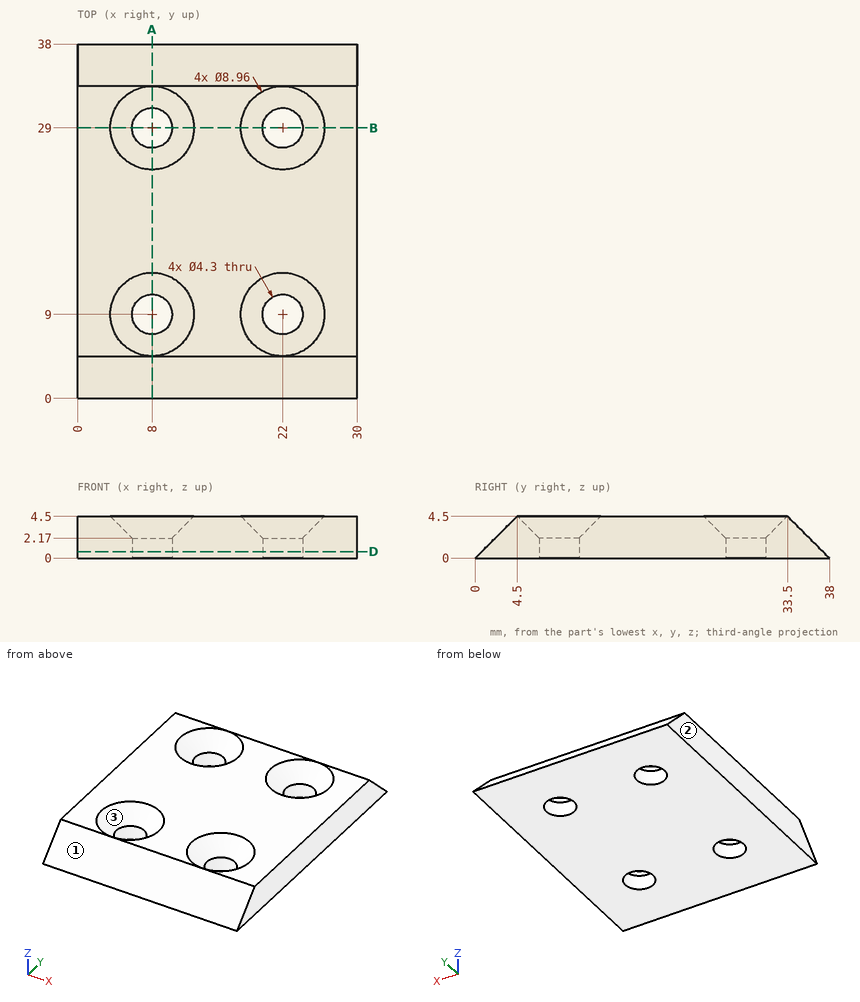
Here's the drawing with two shaded views (mm, measured from the low corner). I have some questions. Round coordinates to 2 decimals unless told otherwise and drop trailing zeros. Loops run counter-clockwise (first coordinate to the right, second up) from the corner with the lowest first, then second, coordinate; pieces in that order, holes last. Notation, with made-up numbers: (-10.5, 41) - (-2.5, 41) arc R15 cw to (-2.5, 54) - close; hole circle Ø2 at (56, 82.5). An arc over 180 degrees is marked (long way). Write item = value, one per line.
1) Imagine slicing it at A-A (x = 8). Give the number of separate pieces and of enclosed holes in the cut face, and give its area (3 significant figures).
Computed:
separate_pieces = 3
enclosed_holes = 0
area = 101 mm2
2) I need wall thicknesses on line 1 along X through (y, z) = (29, 1.4); line 2 along Y through (x, z) = (8, 0.85); line 3 along Y through (x, z) = (23, 3.9). Which ranges of each line are inside material? Lowest first, please. Write a range as from..to.
Computed:
line_1 = 0..5.85, 10.15..19.85, 24.15..30
line_2 = 0.85..6.85, 11.15..26.85, 31.15..37.15
line_3 = 3.9..5.25, 12.75..25.25, 32.75..34.1
3) Imagine slicing it at B-B (y = 29). Please give me the cut outline in (x, z).
Computed:
outline = (0, 0) - (5.85, 0) - (5.85, 2.17) - (3.52, 4.5) - (0, 4.5) - close; (10.15, 0) - (19.85, 0) - (19.85, 2.17) - (17.52, 4.5) - (12.48, 4.5) - (10.15, 2.17) - close; (24.15, 0) - (30, 0) - (30, 4.5) - (26.48, 4.5) - (24.15, 2.17) - close
4) If we mould it in two halves opening along Y, with no side actions, what happens to the marked faces 1, 2 and 3? For each: pulls with the +Y half, pulls with the -Y half, needs draft (parallel to the pull), parting line crosses it, or undercut.
Computed:
face_1 = pulls with the -Y half
face_2 = needs draft
face_3 = undercut
5) Imagine slicing it at D-D (z = 0.7). Please give me the cut outline in (x, y), and give its area (3 significant figures).
Computed:
outline = (0, 0.7) - (30, 0.7) - (30, 37.3) - (0, 37.3) - close; hole circle Ø4.3 at (8, 9); hole circle Ø4.3 at (8, 29); hole circle Ø4.3 at (22, 9); hole circle Ø4.3 at (22, 29)
area = 1,040 mm2
6) I'm going to push a flat-ended pin straight in: P1, Ø5.5, axis at x = 22, y = 29, coming from the +Z side. Where does the tip first touch, or does it pass through?
Computed:
P1 = 2.77
